The listing builds one solid part. Answer for the finished solid, in the listing's coordinates (mm). Round coordinates to 2 decimals unless told otherwise and drop trailing zeros. Write each loop counter-clockwise with the first axis right and the second up, starting at its lowest first coordinate (ties: lowest second). Pieces come first, ordered by that corner, then holes. Notation, with made-up numbers: (30.5, 82.5) - (80.5, 82.5) arc R10 cw to (80.5, 88.5) - close; hole circle Ø2 at (1.25, -27.75). An arc over 180 degrees is marked (long way). Answer as CSV lines item,"result". Start each with the question number.
Item 1: Straight lines are drawn through the part: line 1 along X through (y, z) = (-0.25, -233.5); line 2 along X through (y, z) = (9.55, -280). For each, find the intervals that lie inside material, in ascending order. Write a range as [from, to].
Item 2: A cutting plane is placed at A-A on y = 3.5. Determine the outline of the cut face in (x, z), and give its area (3 significant figures).
Item 3: A cutting plane is placed at B-B on z = -67. Determine the outline of the cut face in (x, y), and give its area (3 significant figures).
Item 4: Flat-ended cylindrical pins translate along their axes: pin 1 (3.5 mm diameter, centred on x = 0, z = 200, fed in from -Y); pin 2 (5 mm diameter, centred on x = 0, z = 107.3, fed in from -Y); pin 3 (6.5 mm diameter, centred on x = 0, z = -90, fed in from -Y); pin 4 (0.5 mm diameter, centred on x = 9.5, z = -79, fed in from -Y). Find the tip coordinate at first contact, or state that the pin passes through.
```python
from build123d import *

# Parameters (mm, degrees)
SKETCH_1_W                       = 20
SKETCH_1_H                       = 20
SKETCH_1_W_2                     = 18
SKETCH_1_H_2                     = 18
EXTRUDE_1_DEPTH                  = 290
HOLE_WIZARD_4_0_4_1_D            = 4
HOLE_WIZARD_4_0_4_2_D            = 4
HOLE_WIZARD_4_0_4_3_D            = 4
HOLE_WIZARD_4_0_4_4_D            = 4
HOLE_WIZARD_4_0_4_6_REACH        = 292.861
HOLE_WIZARD_4_0_4_6_BORE_R       = 2
HOLE_WIZARD_13_0_13_1_D          = 13
HOLE_WIZARD_13_0_13_1_DEPTH      = 1.001
SKETCH_14_W                      = 10
SKETCH_14_H                      = 5
CUT_EXTRUDE_1_DEPTH              = 10
SKETCH_17_R                      = 1
CUT_EXTRUDE_3_DEPTH              = 20
PATTERN_LINEAR_1_COUNT           = 2
PATTERN_LINEAR_1_PITCH           = 10
PATTERN_LINEAR_2_COUNT           = 2
PATTERN_LINEAR_2_PITCH           = 40
PATTERN_LINEAR_2_COPY_1_SKETCH_R = 1
PATTERN_LINEAR_2_COPY_1_DEPTH    = 20
PATTERN_LINEAR_3_COUNT           = 2
PATTERN_LINEAR_3_PITCH           = 160
PATTERN_LINEAR_3_COPY_1_SKETCH_R = 1
PATTERN_LINEAR_3_COPY_1_DEPTH    = 20
HOLE_WIZARD_4_0_4_7_D            = 4


with BuildPart() as part:
    # 草图1 → 凸台-拉伸1 (new, symmetric)
    with BuildSketch(Plane.XY):
        Rectangle(SKETCH_1_W, SKETCH_1_H)
        Rectangle(SKETCH_1_W_2, SKETCH_1_H_2, mode=Mode.SUBTRACT)
    extrude(amount=EXTRUDE_1_DEPTH, both=True)

    # Ø4.0 (4) 直径孔1 (through all)
    with Locations(Plane(origin=(0, 10, 0), x_dir=(1, 0, 0), z_dir=(0, 1, 0))):
        with Locations((0, 155)):
            hole_wizard_4_0_4_1 = Hole(HOLE_WIZARD_4_0_4_1_D / 2)

    # 镜向1: Ø4.0 (4) 直径孔1 across plane
    add(hole_wizard_4_0_4_1.mirror(Plane.XY), mode=Mode.SUBTRACT)

    # Ø4.0 (4) 直径孔2 (through all)
    with Locations(Plane(origin=(0, 10, 0), x_dir=(1, 0, 0), z_dir=(0, 1, 0))):
        with Locations((0, 280)):
            hole_wizard_4_0_4_2 = Hole(HOLE_WIZARD_4_0_4_2_D / 2)

    # 镜向2: Ø4.0 (4) 直径孔2 across plane
    add(hole_wizard_4_0_4_2.mirror(Plane.XY), mode=Mode.SUBTRACT)

    # Ø4.0 (4) 直径孔3 (through all)
    with Locations(Plane(origin=(0, -10, 0), x_dir=(-1, 0, 0), z_dir=(0, -1, 0))):
        with Locations((0, 220), (0, 200)):
            hole_wizard_4_0_4_3 = Hole(HOLE_WIZARD_4_0_4_3_D / 2)

    # Ø4.0 (4) 直径孔4 (through all)
    with Locations(Plane(origin=(0, 10, 0), x_dir=(1, 0, 0), z_dir=(0, 1, 0))):
        with Locations((0, 90)):
            Hole(HOLE_WIZARD_4_0_4_4_D / 2)

    # 镜向3: Ø4.0 (4) 直径孔3 across plane
    add(hole_wizard_4_0_4_3.mirror(Plane.XY), mode=Mode.SUBTRACT)

    # Ø4.0 (4) 直径孔6 bore → Ø4.0 (4) 直径孔6 (cut, up to next)
    with BuildSketch(Plane(origin=(0, 10, 0), x_dir=(1, 0, 0), z_dir=(0, 1, 0)), mode=Mode.PRIVATE) as hole_wizard_4_0_4_6_sk1:
        with Locations((0, 107.3)):
            Circle(HOLE_WIZARD_4_0_4_6_BORE_R)
    hole_wizard_4_0_4_6_tool1 = extrude(hole_wizard_4_0_4_6_sk1.sketch, amount=-HOLE_WIZARD_4_0_4_6_REACH, mode=Mode.PRIVATE) & part.part
    hole_wizard_4_0_4_6 = hole_wizard_4_0_4_6_tool1.solids().sort_by_distance((0, 10, -107.3))[0]
    add(hole_wizard_4_0_4_6, mode=Mode.SUBTRACT)

    # 镜向4: Ø4.0 (4) 直径孔6 across plane
    add(hole_wizard_4_0_4_6.mirror(Plane.XY), mode=Mode.SUBTRACT)

    # Ø13.0 (13) 直径孔1
    with Locations(Plane(origin=(0, -9, 0), x_dir=(1, 0, 0), z_dir=(0, 1, 0))):
        with Locations((0, 107.3)):
            hole_wizard_13_0_13_1 = Hole(HOLE_WIZARD_13_0_13_1_D / 2, depth=HOLE_WIZARD_13_0_13_1_DEPTH)

    # 镜向5: Ø13.0 (13) 直径孔1 across plane
    add(hole_wizard_13_0_13_1.mirror(Plane.XY), mode=Mode.SUBTRACT)

    # 草图14 → 切除-拉伸1 (cut)
    with BuildSketch(Plane.XZ.offset(10)):
        with Locations((-5, -82.5)):
            Rectangle(SKETCH_14_W, SKETCH_14_H)
        with Locations((-5, -77.5)):
            Rectangle(SKETCH_14_W, SKETCH_14_H)
        Polygon((0, -80), (0, -85), (10, -85), (10, -75), (0, -75), align=None)
    cut_extrude_1 = extrude(amount=-CUT_EXTRUDE_1_DEPTH, mode=Mode.SUBTRACT)

    # 草图17 → 切除-拉伸3 (cut)
    with BuildSketch(Plane(origin=(10, 0, 0), x_dir=(0, 0, -1), z_dir=(1, 0, 0))):
        with Locations((85, -1)):
            Circle(SKETCH_17_R)
    cut_extrude_3 = extrude(amount=-CUT_EXTRUDE_3_DEPTH, mode=Mode.SUBTRACT)

    # 阵列(线性)1: 切除-拉伸3 ×2
    with Locations(*[(0, 0, i * PATTERN_LINEAR_1_PITCH) for i in range(1, PATTERN_LINEAR_1_COUNT)]):
        add(cut_extrude_3, mode=Mode.SUBTRACT)

    # 阵列(线性)2: 切除-拉伸1, 切除-拉伸3 ×2
    with Locations(*[(0, 0, i * PATTERN_LINEAR_2_PITCH) for i in range(1, PATTERN_LINEAR_2_COUNT)]):
        add(cut_extrude_1, mode=Mode.SUBTRACT)
        add(cut_extrude_3, mode=Mode.SUBTRACT)

    # 阵列(线性)2 copy 1 sketch → 阵列(线性)2 copy 1 (cut)
    with BuildSketch(Plane(origin=(10, 0, 50), x_dir=(0, 0, -1), z_dir=(1, 0, 0))):
        with Locations((85, -1)):
            Circle(PATTERN_LINEAR_2_COPY_1_SKETCH_R)
    extrude(amount=-PATTERN_LINEAR_2_COPY_1_DEPTH, mode=Mode.SUBTRACT)

    # 阵列(线性)3: 切除-拉伸1, 切除-拉伸3 ×2
    with Locations(*[(0, 0, i * PATTERN_LINEAR_3_PITCH) for i in range(1, PATTERN_LINEAR_3_COUNT)]):
        add(cut_extrude_1, mode=Mode.SUBTRACT)
        add(cut_extrude_3, mode=Mode.SUBTRACT)

    # 阵列(线性)3 copy 1 sketch → 阵列(线性)3 copy 1 (cut)
    with BuildSketch(Plane(origin=(10, 0, 170), x_dir=(0, 0, -1), z_dir=(1, 0, 0))):
        with Locations((85, -1)):
            Circle(PATTERN_LINEAR_3_COPY_1_SKETCH_R)
    extrude(amount=-PATTERN_LINEAR_3_COPY_1_DEPTH, mode=Mode.SUBTRACT)

    # Ø4.0 (4) 直径孔7 (through all)
    with Locations(Plane(origin=(0, -10, 0), x_dir=(-1, 0, 0), z_dir=(0, -1, 0))):
        with Locations((0, 0)):
            Hole(HOLE_WIZARD_4_0_4_7_D / 2)


solid = part.part
```
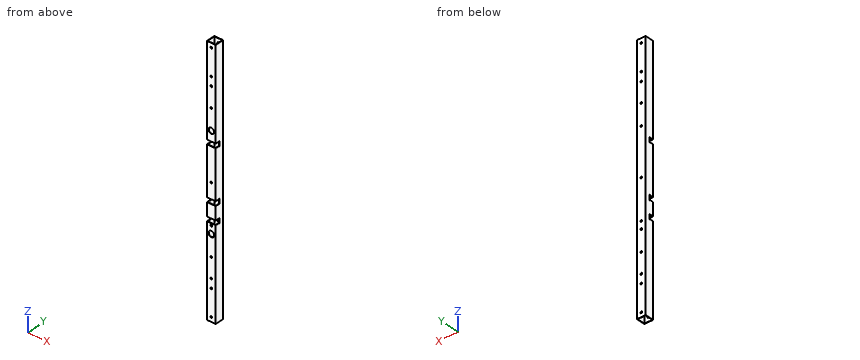
Geometry says:
1,line 1,"x = [-10, -9], [9, 10]"
1,line 2,"x = [-10, -2], [2, 10]"
2,outline,"(-10, -290) - (-9, -290) - (-9, 290) - (-10, 290) - close; (9, -290) - (10, -290) - (10, 290) - (9, 290) - close"
2,area,"1,160 mm^2"
3,outline,"(-10, -10) - (10, -10) - (10, 10) - (-10, 10) - close; hole (-9, -9) - (9, -9) - (9, 9) - (-9, 9) - close"
3,area,"76.0 mm^2"
4,pin 1,"passes through"
4,pin 2,"stops at y = 9"
4,pin 3,"stops at y = -10"
4,pin 4,"stops at y = 0"
